For this review, take the finished solid that the model builds, in its own axes (mm). Give positions to 0.01 mm unless a question says otherwise; leave off trailing zeros. Order: outer loops, then holes, each group sorted by start corner. A loop starts at its lowest first (then second) coordinate and runs counter-clockwise, first axis right, second up. Notation, with made-up numbers: (9, -13.75) - (62, -13.75) arc R21 cw to (62, 21.25) - close; hole circle Ø9 at (73, 86). An arc over 180 degrees is marked (long way). One line per item, written item: value.
```python
from build123d import *

# Parameters (mm, degrees)
CROQUIS1_W              = 450
CROQUIS1_H              = 275
SALIENTE_EXTRUIR1_DEPTH = 65
REDONDEO1_R             = 70
REDONDEO2_R             = 70
REDONDEO3_R             = 50


with BuildPart() as part:
    # Croquis1 → Saliente-Extruir1 (new body)
    with BuildSketch(Plane.XY):
        Rectangle(CROQUIS1_W, CROQUIS1_H)
    extrude(amount=SALIENTE_EXTRUIR1_DEPTH)

    # Redondeo1
    redondeo1_edges = [part.edges().sort_by_distance(p)[0] for p in [
        (-225, -137.5, 32.5),
    ]]
    fillet(redondeo1_edges, radius=REDONDEO1_R)

    # Redondeo2
    redondeo2_edges = [part.edges().sort_by_distance(p)[0] for p in [
        (225, -137.5, 32.5),
    ]]
    fillet(redondeo2_edges, radius=REDONDEO2_R)

    # Redondeo3
    redondeo3_edges = [part.edges().sort_by_distance(p)[0] for p in [
        (0, -137.5, 65),
        (-225, 35, 65),
        (-204.497474683, -116.997474683, 65),
        (225, 35, 65),
        (204.497474683, -116.997474683, 65),
    ]]
    fillet(redondeo3_edges, radius=REDONDEO3_R)


solid = part.part
```
(1) Take a section at A-A (x = -127.5). Write out the cut boundary in (y, z), then the cut area to 3 significant figures.
Answers below:
outline: (-137.5, 0) - (137.5, 0) - (137.5, 65) - (-87.5, 65) arc R50 ccw to (-137.5, 15) - close
area: 17,300 mm^2
(2) For P1, Ø10, axis at y = 84.5, z = 52.5, coming from the +X side; P2, Ø1, axis at x = 156, z = 17.5, coming from the -Y side, all flat-tipped, find the tip position at first contact; note any pin that passes through.
Answers below:
P1: stops at x = 213
P2: stops at y = -137.45
(3) Take a section at C-C (z = 10). Write out the cut boundary in (x, y), then the cut area to 3 significant figures.
Answers below:
outline: (-225, -67.5) arc R70 ccw to (-155, -137.5) - (155, -137.5) arc R70 ccw to (225, -67.5) - (225, 137.5) - (-225, 137.5) - close
area: 122,000 mm^2
(4) Wall thickness on line 1 (Z direction, x = -203, y = -70); line 2 (X direction, y = 40, z = 61); line 3 (Y direction, x = -185, z = 29): over which ranges is each line inside the solid? List them lowest first. Write a range as from..to.
Answers below:
line 1: z = 0..56.38
line 2: x = -194.6..194.6
line 3: y = -128.52..137.5
(5) Draft analysis for pull direction Z (two halves, no side actions). For faces 1 (the face through (-3, 2, 0)), 2 (the face through (-205.04, -116.45, 7.61)), 3 (the face through (210.742, 36.435, 49.964)), state which applies: pulls with the +Z half, pulls with the -Z half, needs draft (parallel to the pull), parting line crosses it, or undercut.
Answers below:
face 1: pulls with the -Z half
face 2: needs draft
face 3: pulls with the +Z half
(6) Take a section at B-B (y = -62). Write out the cut boundary in (x, z), then the cut area to 3 significant figures.
Answers below:
outline: (-225, 0) - (225, 0) - (225, 15) arc R50 ccw to (175, 65) - (-175, 65) arc R50 ccw to (-225, 15) - close
area: 28,200 mm^2
